Here's how the part is built. I have some questions about the finished solid (model axes, mm). Face numbers are marked on the shaded views. Round coordinates to 2 decimals unless told otherwise and drop trailing zeros. Order: outer loops, then holes, each group sorted by start corner. A loop starts at its lowest first (then second) coordinate and runs counter-clockwise, first axis right, second up.
```python
from build123d import *
from OCP.BRepFilletAPI import BRepFilletAPI_MakeChamfer

# Parameters (mm, degrees)
SKETCH5_W             = 90
SKETCH5_H             = 67.5
SKETCH5_W_2           = 85
SKETCH5_H_2           = 62.5
BOSS_EXTRUDE3_DEPTH   = 10
FILLET1_R             = 3
SKETCH7_R             = 3.3
SKETCH7_R_2           = 1.3
BOSS_EXTRUDE5_DEPTH   = 8.5
SKETCH11_W            = 10
SKETCH11_H            = 4
BOSS_EXTRUDE6_DEPTH   = 12
FILLET3_R             = 3
SKETCH13_R            = 2.25
CUT_EXTRUDE1_DEPTH    = 113.659886384
CHAMFER2_SIZE         = 1
CHAMFER2_SIZE2        = 1.732050808
CIRPATTERN1_OUTLINE_R = 2.25
CIRPATTERN1_DEPTH     = 2.9999999
CIRPATTERN1_START     = 2.9999999
CIRPATTERN1_2_DEPTH   = 1.0000001
FILLET5_R             = 3


with BuildPart() as part:
    # Sketch5 → Boss-Extrude3 (new body)
    with BuildSketch(Plane(origin=(0, 0, 0), x_dir=(1, 0, 0), z_dir=(0, 1, 0))):
        with Locations((45, 33.75)):
            Rectangle(SKETCH5_W, SKETCH5_H)
        with Locations((45, 33.75)):
            Rectangle(SKETCH5_W_2, SKETCH5_H_2, mode=Mode.SUBTRACT)
    extrude(amount=BOSS_EXTRUDE3_DEPTH)

    # Fillet1
    fillet1_edges = [part.edges().sort_by_distance(p)[0] for p in [
        (87.5, 5, -2.5),
        (87.5, 5, -65),
        (2.5, 5, -65),
        (2.5, 5, -2.5),
        (90, 5, -67.5),
        (90, 5, 0),
        (0, 5, 0),
        (0, 5, -67.5),
    ]]
    fillet(fillet1_edges, radius=FILLET1_R)

    # Sketch7 → Boss-Extrude5 (add)
    # profile 1 of 4: a face of its own
    with BuildSketch(Plane(origin=(0, 0, 0), x_dir=(1, 0, 0), z_dir=(0, 1, 0))):
        with Locations((5.63, 5.81)):
            Circle(SKETCH7_R)
        with Locations(Location((5.63, 5.81, 0), (0, 0, 270))):
            Circle(SKETCH7_R_2, mode=Mode.SUBTRACT)
    # profile 2 of 4: a face of its own
    with BuildSketch(Plane(origin=(0, 0, 0), x_dir=(1, 0, 0), z_dir=(0, 1, 0))):
        with Locations((5.63, 61.69)):
            Circle(SKETCH7_R)
        with Locations(Location((5.63, 61.69, 0), (0, 0, 270))):
            Circle(SKETCH7_R_2, mode=Mode.SUBTRACT)
    # profile 3 of 4: a face of its own
    with BuildSketch(Plane(origin=(0, 0, 0), x_dir=(1, 0, 0), z_dir=(0, 1, 0))):
        with Locations((84.37, 5.81)):
            Circle(SKETCH7_R)
        with Locations(Location((84.37, 5.81, 0), (0, 0, 270))):
            Circle(SKETCH7_R_2, mode=Mode.SUBTRACT)
    # profile 4 of 4: a face of its own
    with BuildSketch(Plane(origin=(0, 0, 0), x_dir=(1, 0, 0), z_dir=(0, 1, 0))):
        with Locations((84.37, 61.69)):
            Circle(SKETCH7_R)
        with Locations(Location((84.37, 61.69, 0), (0, 0, 270))):
            Circle(SKETCH7_R_2, mode=Mode.SUBTRACT)
    extrude(amount=BOSS_EXTRUDE5_DEPTH)

    # Sketch11 → Boss-Extrude6 (add)
    with BuildSketch(Plane.XY):
        with Locations((11.5, 2)):
            Rectangle(SKETCH11_W, SKETCH11_H)
        with Locations((78.5, 2)):
            Rectangle(SKETCH11_W, SKETCH11_H)
    extrude(amount=BOSS_EXTRUDE6_DEPTH)

    # Fillet3
    fillet3_edges = [part.edges().sort_by_distance(p)[0] for p in [
        (6.5, 2, 0),
        (16.5, 2, 0),
        (11.5, 4, 0),
        (6.5, 2, 12),
        (16.5, 2, 12),
        (73.5, 2, 0),
        (83.5, 2, 0),
        (78.5, 4, 0),
        (73.5, 2, 12),
        (83.5, 2, 12),
    ]]
    fillet(fillet3_edges, radius=FILLET3_R)

    # Sketch13 → Cut-Extrude1 (cut, through all)
    with BuildSketch(Plane(origin=(0, 4, 0), x_dir=(1, 0, 0), z_dir=(0, 1, 0))):
        with Locations(Location((11.5, -7, 0), (0, 0, 270))):
            Circle(SKETCH13_R)
        with Locations(Location((78.5, -7, 0), (0, 0, 270))):
            Circle(SKETCH13_R)
    extrude(amount=-CUT_EXTRUDE1_DEPTH, mode=Mode.SUBTRACT)

    # Chamfer2: one chamfer whose edges measure the first distance from different faces: ONE call of the kernel's chamfer builder (chamfer() names one face for all edges)
    chamfer2_edges_1 = [part.edges().sort_by_distance(p)[0] for p in [
        (11.5, 4, 4.75),
    ]]
    chamfer2_side_1 = [part.faces().sort_by_distance(p)[0] for p in [
        (11.5, 2, 4.75),
    ]]
    chamfer2_edges_2 = [part.edges().sort_by_distance(p)[0] for p in [
        (78.5, 4, 4.75),
    ]]
    chamfer2_side_2 = [part.faces().sort_by_distance(p)[0] for p in [
        (78.5, 2, 4.75),
    ]]
    chamfer2 = BRepFilletAPI_MakeChamfer(part.part.solid().wrapped)
    for e in chamfer2_edges_1:
        chamfer2.Add(CHAMFER2_SIZE, CHAMFER2_SIZE2, e.wrapped, chamfer2_side_1[0].wrapped)  # the first distance lies on this face
    for e in chamfer2_edges_2:
        chamfer2.Add(CHAMFER2_SIZE, CHAMFER2_SIZE2, e.wrapped, chamfer2_side_2[0].wrapped)  # the first distance lies on this face
    add(Compound.cast(chamfer2.Shape()), mode=Mode.REPLACE)

    # CirPattern1: read off the stored shape, not the designer's step
    # CirPattern1 outline → CirPattern1 (add)
    # profile 1 of 2: a face of its own
    with BuildSketch(Plane(origin=(0, 0, 0), x_dir=(1, 0, 0), z_dir=(0, 1, 0))):
        with BuildLine():
            Line((73.5, 76.5), (73.5, 67.5))
            Line((73.5, 67.5), (83.5, 67.5))
            Line((83.5, 67.5), (83.5, 76.5))
            ThreePointArc((83.5, 76.5), (82.621320344, 78.621320344), (80.5, 79.5))
            Line((80.5, 79.5), (76.5, 79.5))
            ThreePointArc((76.5, 79.5), (74.378679656, 78.621320344), (73.5, 76.5))
        make_face()
        with Locations((78.5, 74.5)):
            Circle(CIRPATTERN1_OUTLINE_R, mode=Mode.SUBTRACT)
    # profile 2 of 2: a face of its own
    with BuildSketch(Plane(origin=(0, 0, 0), x_dir=(1, 0, 0), z_dir=(0, 1, 0))):
        with BuildLine():
            Line((6.5, 76.5), (6.5, 67.5))
            Line((6.5, 67.5), (16.5, 67.5))
            Line((16.5, 67.5), (16.5, 76.5))
            ThreePointArc((16.5, 76.5), (15.621320344, 78.621320344), (13.5, 79.5))
            Line((13.5, 79.5), (9.5, 79.5))
            ThreePointArc((9.5, 79.5), (7.378679656, 78.621320344), (6.5, 76.5))
        make_face()
        with Locations((11.5, 74.5)):
            Circle(CIRPATTERN1_OUTLINE_R, mode=Mode.SUBTRACT)
    extrude(amount=CIRPATTERN1_DEPTH)

    # CirPattern1 2 outline → CirPattern1 2 (add)
    with BuildSketch(Plane(origin=(0, 0, 0), x_dir=(1, 0, 0), z_dir=(0, 1, 0)).offset(CIRPATTERN1_START)):
        with BuildLine():
            Line((73.5, 76.5), (73.5, 67.5))
            Line((73.5, 67.5), (83.5, 67.5))
            Line((83.5, 67.5), (83.5, 76.5))
            ThreePointArc((83.5, 76.5), (82.621320344, 78.621320344), (80.5, 79.5))
            Line((80.5, 79.5), (76.5, 79.5))
            ThreePointArc((76.5, 79.5), (74.378679656, 78.621320344), (73.5, 76.5))
        make_face()
        with BuildLine():
            Line((6.5, 76.5), (6.5, 67.5))
            Line((6.5, 67.5), (16.5, 67.5))
            Line((16.5, 67.5), (16.5, 76.5))
            ThreePointArc((16.5, 76.5), (15.621320344, 78.621320344), (13.5, 79.5))
            Line((13.5, 79.5), (9.5, 79.5))
            ThreePointArc((9.5, 79.5), (7.378679656, 78.621320344), (6.5, 76.5))
        make_face()
    extrude(amount=CIRPATTERN1_2_DEPTH)

    # CirPattern1 3: loft between two sections, ruled curve by curve
    cirpattern1_3_from = [
        Edge.make_three_point_arc((11.5, 3, -76.75), (9.25, 3, -74.5), (11.5, 3, -72.25)),
        Edge.make_three_point_arc((11.5, 3, -72.25), (13.75, 3, -74.5), (11.5, 3, -76.75)),
    ]
    cirpattern1_3_to = [
        Edge.make_three_point_arc((11.5, 4, -78.482050808), (7.517949192, 4, -74.5), (11.5, 4, -70.517949192)),
        Edge.make_three_point_arc((11.5, 4, -70.517949192), (15.482050808, 4, -74.5), (11.5, 4, -78.482050808)),
    ]
    cirpattern1_3 = Solid(Shell([*[Face.make_surface_from_curves(cirpattern1_3_from[k], cirpattern1_3_to[k]) for k in range(2)], Face(Wire(cirpattern1_3_from)), Face(Wire(cirpattern1_3_to))]))
    add(cirpattern1_3, mode=Mode.SUBTRACT)

    # CirPattern1 4: loft between two sections, ruled curve by curve
    cirpattern1_4_from = [
        Edge.make_three_point_arc((78.5, 3, -76.75), (76.25, 3, -74.5), (78.5, 3, -72.25)),
        Edge.make_three_point_arc((78.5, 3, -72.25), (80.75, 3, -74.5), (78.5, 3, -76.75)),
    ]
    cirpattern1_4_to = [
        Edge.make_three_point_arc((78.5, 4, -78.482050808), (74.517949192, 4, -74.5), (78.5, 4, -70.517949192)),
        Edge.make_three_point_arc((78.5, 4, -70.517949192), (82.482050808, 4, -74.5), (78.5, 4, -78.482050808)),
    ]
    cirpattern1_4 = Solid(Shell([*[Face.make_surface_from_curves(cirpattern1_4_from[k], cirpattern1_4_to[k]) for k in range(2)], Face(Wire(cirpattern1_4_from)), Face(Wire(cirpattern1_4_to))]))
    add(cirpattern1_4, mode=Mode.SUBTRACT)

    # Fillet5
    fillet5_edges = [part.edges().sort_by_distance(p)[0] for p in [
        (83.5, 2, -67.5),
        (73.5, 2, -67.5),
        (78.5, 4, -67.5),
        (16.5, 2, -67.5),
        (6.5, 2, -67.5),
        (11.5, 4, -67.5),
    ]]
    fillet(fillet5_edges, radius=FILLET5_R)


solid = part.part
```
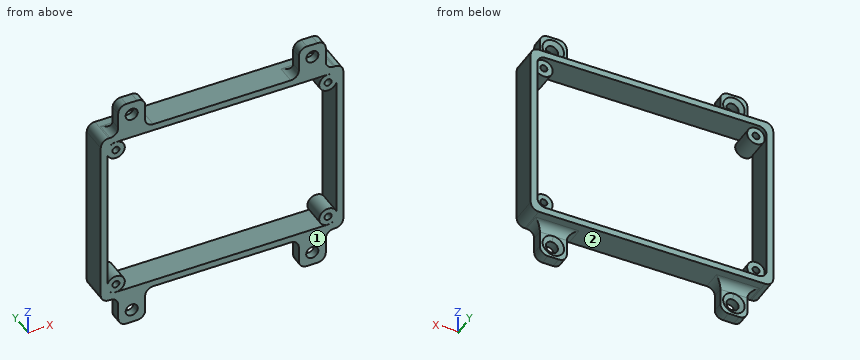
1. I'm going to push flat-ended pins straight in: P1, Ø2.5, axis at x = 13, z = -74, coming from the +Y side; P2, Ø6, axis at y = 7, z = -69, coming from the -X side; P3, Ø1, axis at x = 48, y = 1.5, coming from the +Z side; P4, Ø5, axis at x = 78.5, z = -74.5, coming from the -Y side. Where does each tip first touch, or does it pass through?
Evaluation:
P1: stops at y = 3.34
P2: stops at x = 0.4
P3: stops at z = 0
P4: stops at y = 0
2. If we section it at C-C, the plane y = 5.5: State how many separate pieces and enclosed holes the cut face has, and give its area (3 significant figures).
Evaluation:
separate pieces: 1
enclosed holes: 5
area: 899 mm2
3. If we section it at B-B, the plane z = 7: Write out the boundary of the cut face in (x, y), and give its area (3 significant figures).
Evaluation:
outline: (6.5, 0) - (9.25, 0) - (9.25, 3) - (7.52, 4) - (6.5, 4) - close; (13.75, 0) - (16.5, 0) - (16.5, 4) - (15.48, 4) - (13.75, 3) - close; (73.5, 0) - (76.25, 0) - (76.25, 3) - (74.52, 4) - (73.5, 4) - close; (80.75, 0) - (83.5, 0) - (83.5, 4) - (82.48, 4) - (80.75, 3) - close
area: 40.5 mm2
4. If we mould it in two halves opening along X, with no side actions, what happens to the marked faces 1 and 2? For each: released by +X, released by -X, zero draft, split by the parting line, or undercut.
Evaluation:
face 1: zero draft
face 2: undercut
5. I need wall thicknesses on probe 1 along X at (y, z) = (0.8, -74.5); probe 2 along X at (y, z) = (4, -50.5); probe 3 along Z at (x, y) = (28, 9). Which ranges of each line are inside material? Lowest first, please.
Evaluation:
probe 1: x = 6.5 to 9.25, 13.75 to 16.5, 73.5 to 76.25, 80.75 to 83.5
probe 2: x = 0 to 2.5, 87.5 to 90
probe 3: z = -67.5 to -65, -2.5 to 0
6. If we section it at A-A, the plane x = 41: Write out the boundary of the cut face in (y, z).
Evaluation:
outline: (0, -67.5) - (10, -67.5) - (10, -65) - (0, -65) - close; (0, -2.5) - (10, -2.5) - (10, 0) - (0, 0) - close
